For this review, take the finished solid that the model builds, in its own axes (mm). Face numbers are marked on the shaded views. A direction names the side the tool comes from. Round coordinates to 2 decimals unless told otherwise and drop trailing zeros. Write each loop counter-clockwise with the first axis right and the second up, starting at its lowest first coordinate (ties: lowest second). Pieces come first, ordered by that corner, then holes. Notation, with made-up numbers: M 19,26.5 L 76,26.5 A20 cw 76,40.5 Z; hole C -39,89.5 d9. An arc over 180 degrees is marked long. Use one line per item in the form item = value. Start each with the question number.
Item 1: Draft analysis for pull direction X (two halves, no side actions). For the marked faces 4, 5, 6 and 7, state which applies: released by +X, released by -X, zero draft, split by the parting line, or undercut.
Item 2: Add section D-D (x = -55). Count the separate pieces of the cut face and the enclosed holes in it, and give its area (3 significant figures).
Item 3: For line 1 (Y direction, x = -55, z = -110); line 2 (X direction, y = 8, z = -17); line 3 (Y direction, x = -76, z = -78.5), list the stretches that pass through material, from the lowest coordinate up. Write a range as [from, to].
Item 4: Add section C-C (z = -90.5). State the section outline as (x, y) points, and give its area (3 significant figures).
Item 5: Add section B-B (x = -90). State the section outline as (y, z) points (3 decimals).
Item 6: Add section A-A (z = -17). State the section outline as (x, y) points, and give its area (3 significant figures).
Item 7: For P1, Ø5, axis at y = 81.5, z = -108, coming from the +X side; P2, Ø2.5, axis at x = -102, y = 7, coming from the -Z side; P3, Ø7, axis at x = -15.5, z = -15, coming from the +Y side, all flat-tipped, find the tip position at first contact; note any pin that passes through.
Item 8: For the marked faces 1, 2 and 3, list the 3-axis set-ups (+Z, -Z, +X, -X, +Y, -Y) from which the entire face can be reached by the end or side of a thin tool; tool diameter is ignored.
from build123d import *

# Parameters (mm, degrees)
SKETCH1_R           = 11.5
BOSS_EXTRUDE1_DEPTH = 14
SKETCH1_3_R         = 11.5
SKETCH1_3_R_2       = 6
BOSS_EXTRUDE2_DEPTH = 19
BOSS_EXTRUDE3_DEPTH = 4
SKETCH8_R           = 10
BOSS_EXTRUDE4_DEPTH = 11
FILLET1_R           = 10
FILLET2_R           = 16
FILLET10_R          = 5
FILLET8_R           = 4
FILLET9_START       = -43
FILLET9_DEPTH       = 13


with BuildPart() as part:
    # Sketch1 → Boss-Extrude1 (new body)
    with BuildSketch(Plane(origin=(0, 0, 0), x_dir=(1, 0, 0), z_dir=(0, 1, 0))):
        with BuildLine():
            Line((-77, 64), (-77, 97))
            ThreePointArc((-77, 97), (-55, 119), (-33, 97))
            Line((-33, 97), (-33, 64))
            ThreePointArc((-33, 64), (-27.142135624, 49.857864376), (-13, 44))
            Line((-13, 44), (-5, 44))
            ThreePointArc((-5, 44), (-1.464466094, 42.535533906), (0, 39))
            Line((0, 39), (0, 5))
            ThreePointArc((0, 5), (-1.464466094, 1.464466094), (-5, 0))
            Line((-5, 0), (-105, 0))
            ThreePointArc((-105, 0), (-108.535533906, 1.464466094), (-110, 5))
            Line((-110, 5), (-110, 39))
            ThreePointArc((-110, 39), (-108.535533906, 42.535533906), (-105, 44))
            Line((-105, 44), (-97, 44))
            ThreePointArc((-97, 44), (-82.857864376, 49.857864376), (-77, 64))
        make_face()
        with Locations(Location((-20, 17, 0), (0, 0, 270))):
            Circle(SKETCH1_R, mode=Mode.SUBTRACT)
        with Locations(Location((-90, 17, 0), (0, 0, 270))):
            Circle(SKETCH1_R, mode=Mode.SUBTRACT)
        with BuildLine():
            Line((-45, 97), (-45, 77))
            ThreePointArc((-45, 77), (-55, 67), (-65, 77))
            Line((-65, 77), (-65, 97))
            ThreePointArc((-65, 97), (-55, 107), (-45, 97))
        make_face(mode=Mode.SUBTRACT)
    extrude(amount=BOSS_EXTRUDE1_DEPTH)

    # Sketch1<3> → Boss-Extrude2 (add)
    # profile 1 of 2: a face of its own
    with BuildSketch(Plane(origin=(0, 0, 0), x_dir=(1, 0, 0), z_dir=(0, 1, 0))):
        with Locations(Location((-90, 17, 0), (0, 0, 270))):
            Circle(SKETCH1_3_R)
        with Locations(Location((-90, 17, 0), (0, 0, 270))):
            Circle(SKETCH1_3_R_2, mode=Mode.SUBTRACT)
    # profile 2 of 2: a face of its own
    with BuildSketch(Plane(origin=(0, 0, 0), x_dir=(1, 0, 0), z_dir=(0, 1, 0))):
        with Locations(Location((-20, 17, 0), (0, 0, 270))):
            Circle(SKETCH1_3_R)
        with Locations(Location((-20, 17, 0), (0, 0, 270))):
            Circle(SKETCH1_3_R_2, mode=Mode.SUBTRACT)
    extrude(amount=BOSS_EXTRUDE2_DEPTH)

    # Sketch3 → Loft1 section 0
    with BuildSketch(Plane(origin=(0, 73, 0), x_dir=(1, 0, 0), z_dir=(0, 1, 0))):
        with BuildLine():
            Line((-77, 43), (-33, 43))
            Line((-33, 43), (-33, 30))
            Line((-33, 30), (-77, 30))
            Line((-77, 30), (-77, 43))
        make_face()
    # Sketch2 → Loft1 section 1
    with BuildSketch(Plane(origin=(0, 14, 0), x_dir=(1, 0, 0), z_dir=(0, 1, 0))):
        with BuildLine():
            Line((-80, 43), (-30, 43))
            Line((-30, 43), (-30, 30))
            Line((-30, 30), (-80, 30))
            Line((-80, 30), (-80, 43))
        make_face()
    loft()

    # Sketch4 → Boss-Extrude3 (add, symmetric)
    with BuildSketch(Plane(origin=(-55, 0, 0), x_dir=(0, 0, -1), z_dir=(1, 0, 0))):
        Polygon((30, 64), (5, 14), (30, 14), align=None)
    extrude(amount=BOSS_EXTRUDE3_DEPTH, both=True)

    # Sketch7 → Loft2 section 0
    with BuildSketch(Plane(origin=(0, 0, -43), x_dir=(-1, 0, 0), z_dir=(0, 0, -1))):
        with BuildLine():
            Line((77, 73), (77.661016949, 60))
            Line((77.661016949, 60), (32.338983051, 60))
            Line((32.338983051, 60), (33, 73))
            Line((33, 73), (77, 73))
        make_face()
    # Sketch6 → Loft2 section 1
    with BuildSketch(Plane.XY.offset(-114)):
        with BuildLine():
            Line((-77, 73), (-77.661016949, 60))
            Line((-77.661016949, 60), (-32.338983051, 60))
            Line((-32.338983051, 60), (-33, 73))
            Line((-33, 73), (-77, 73))
        make_face()
    loft()

    # Sketch8 → Boss-Extrude4 (add)
    with BuildSketch(Plane.XY.offset(-114)):
        with BuildLine():
            Line((-77, 73), (-77, 96))
            ThreePointArc((-77, 96), (-55, 118), (-33, 96))
            Line((-33, 96), (-33, 73))
            Line((-33, 73), (-77, 73))
        make_face()
        with Locations((-55, 96)):
            Circle(SKETCH8_R, mode=Mode.SUBTRACT)
    extrude(amount=BOSS_EXTRUDE4_DEPTH)

    # Fillet1
    # the kernel refuses this fillet: 10 mm, written as the material it adds along each edge
    with BuildSketch(Plane(origin=(-59, 14, -5), x_dir=(0, 0, 1), z_dir=(1, 0, 0))) as fillet1_piece_1:
        with BuildLine():
            CenterArc((6.217538244, -9.925603288), FILLET1_R, 96.993331588, 56.441617235)
            Line((-2.726733666, -5.453467333), (-2.905619105, -5.364024614))
            Line((-2.905619105, -5.364024614), (-0.178885438, 0.089442719))
            Line((-0.178885438, 0.089442719), (0, 0.2))
            ThreePointArc((0, 0.2), (2.5, 0.2), (4.975649235, 0.198512066))
            Line((4.975649235, 0.198512066), (5, 0))
        make_face()
    extrude(amount=8)

    # Fillet2
    fillet2_edges = [part.edges().sort_by_distance(p)[0] for p in [
        (-55, 64, -30),
    ]]
    fillet(fillet2_edges, radius=FILLET2_R)

    # Fillet10
    fillet10_edges = [part.edges().sort_by_distance(p)[0] for p in [
        (-55, 60, -43),
        (-55, 73, -103),
        (-55, 73, -30),
    ]]
    fillet(fillet10_edges, radius=FILLET10_R)

    # Fillet8
    fillet8_edges = [part.edges().sort_by_distance(p)[0] for p in [
        (-90, 14, -28.5),
        (-20, 14, -28.5),
    ]]
    fillet(fillet8_edges, radius=FILLET8_R)

    # Fillet9: read off the stored shape, not the designer's step
    # Fillet9 outline → Fillet9 (add)
    with BuildSketch(Plane.XY.offset(FILLET9_START)):
        with BuildLine():
            Line((-80, 14), (-79.710408023, 19.695308884))
            ThreePointArc((-79.710408023, 19.695308884), (-81.56915401, 15.650968689), (-85.702666639, 14))
            Line((-85.702666639, 14), (-80, 14))
        make_face()
        with BuildLine():
            Line((-30.289591977, 19.695308884), (-30, 14))
            Line((-30, 14), (-24.297333361, 14))
            ThreePointArc((-24.297333361, 14), (-28.43084599, 15.650968689), (-30.289591977, 19.695308884))
        make_face()
    extrude(amount=FILLET9_DEPTH)


solid = part.part
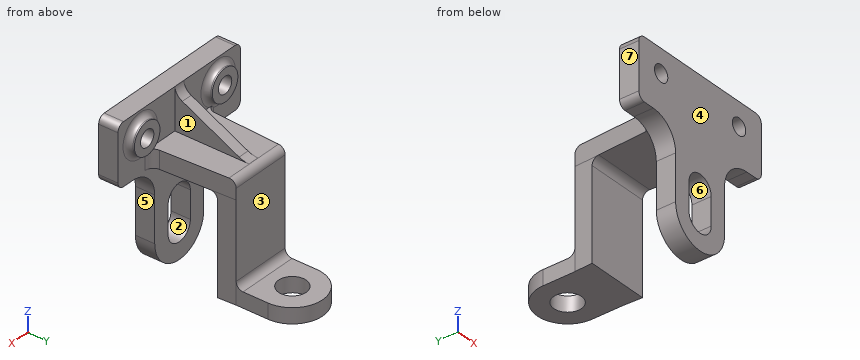
Calculated:
q1.face_4 = zero draft
q1.face_5 = released by +X
q1.face_6 = undercut
q1.face_7 = released by -X
q2.separate_pieces = 3
q2.enclosed_holes = 0
q2.area = 3,710 mm^2
q3.line_1 = [0, 14], [60, 86], [106, 118]
q3.line_2 = [-110, -96], [-84, -26], [-14, 0]
q3.line_3 = [0, 14], [60, 73]
q4.outline = M -77.66,60 L -32.34,60 L -33,73 L -77,73 Z; M -77,0 L -65,0 L -65,14 L -77,14 Z; M -45,0 L -33,0 L -33,14 L -45,14 Z
q4.area = 917 mm^2
q5.outline = M 0,-45.265 L 14,-45.265 L 14,-32.5 A4 cw 18,-28.5 L 19,-28.5 L 19,-23 L 0,-23 Z; M 0,-11 L 19,-11 L 19,-5.5 L 18,-5.5 A4 cw 14,-1.5 L 14,0 L 0,0 Z
q6.outline = M -110,0 L -96,0 L -96,19 L -101.5,19 L -101.5,18 A4 cw -105.5,14 L -110,14 Z; M -84,0 L -26,0 L -26,19 L -31.5,19 L -31.5,18 A4 cw -35.5,14 L -51,14 L -51,38 L -59,38 L -59,14 L -74.5,14 A4 cw -78.5,18 L -78.5,19 L -84,19 Z; M -14,0 L 0,0 L 0,14 L -4.5,14 A4 cw -8.5,18 L -8.5,19 L -14,19 Z
q6.area = 1,520 mm^2
q7.P1 = -33
q7.P2 = -44
q7.P3 = 19
q8.face_1 = +Z, +Y
q8.face_2 = -Y
q8.face_3 = +Z, +X, -X, +Y
